Verification items for the finished model (mm, model axes). A direction names the side the tool comes from. Coordinates: 2 decimals unless noted, no trailing zeros. Order: outer loops, then holes, each group sorted by start corner. A loop starts at its lowest first (then second) coordinate and runs counter-clockwise, first axis right, second up. Notation, with made-up numbers: (86, 29.25) -> (102, 29.25) arc R25 cw to (102, 61.25) -> close; hole circle Ø8 at (-19.5, -10.5). An arc over 180 degrees is marked (long way). Answer as CSV lines item,"result".
```python
from build123d import *

# Parameters (mm, degrees)
BOSS_EXTRUDE1_DEPTH = 79.502
SKETCH2_RX          = 34.87252212
SKETCH2_RY          = 7.136819482
BOSS_EXTRUDE2_DEPTH = 79.502


with BuildPart() as part:
    # Sketch1 → Boss-Extrude1 (new body)
    with BuildSketch(Plane.XY):
        Polygon((0, 0), (101.6, 0), (152.4, 80.572467382), (0, 80.572467382), align=None)
    extrude(amount=BOSS_EXTRUDE1_DEPTH)

    # Sketch2 → Boss-Extrude2 (add)
    with BuildSketch(Plane(origin=(0, 80.572467382, 0), x_dir=(1, 0, 0), z_dir=(0, 1, 0))):
        with Locations(Location((57.268893284, -43.52674359), (0, 0, 21.757695584))):
            Ellipse(SKETCH2_RX, SKETCH2_RY)
    extrude(amount=BOSS_EXTRUDE2_DEPTH)


solid = part.part
```
Item 1: Tool access check on faces 1 (the flat face through (77, 80.572, 48)), 2 (the flat face through (0, 41, 39)). Record the directions out of +Z, -Z, +X, -X, +Y, -Y that give a thin tool (end or side, any length) a straight path to the whole face; none if there is none.
Answer list:
face 1,"+Y"
face 2,"+Z, -Z, -X, +Y, -Y"
Item 2: Depth check by flat-ended pin: pin 1 Ø6 at (y, z) = (83, 51) entering from -X; pin 2 Ø1.5 at (x, z) = (23.5, 51) entering from +Y; pin 3 Ø8 at (y, z) = (36, 38) entering from +X; pin 4 Ø12 at (x, z) = (137, 66.5) entering from -Y. Enter the tip coordinate at first touch or a pass-through.
Answer list:
pin 1,"x = 0"
pin 2,"y = 80.57"
pin 3,"x = 126.82"
pin 4,"y = 46.63"
Item 3: Section check B-B, the plane z = 74. Record the boundary of the cut face in (x, y).
Answer list:
outline,"(0, 0) -> (101.6, 0) -> (152.4, 80.57) -> (0, 80.57) -> close"
Item 4: Section check A-A, the plane x = 17. Record the boundary of the cut face in (y, z).
Answer list:
outline,"(0, 0) -> (80.57, 0) -> (80.57, 79.5) -> (0, 79.5) -> close"
Item 5: Thickness scan on line 1 (Y direction, x = 68.5, z = 8.5); line 2 (X direction, y = 123, z = 40); line 3 (X direction, y = 30, z = 49). Record the ranges inside material, lowest first.
Answer list:
line 1,"0 to 80.57"
line 2,"47.35 to 80.59"
line 3,"0 to 120.51"
